The model under review builds one solid part; all positions refer to its coordinate system, in mm. A direction names the side the tool comes from. Give positions to 0.01 mm unless a question says otherwise; leave off trailing zeros. Write each loop counter-clockwise with the first axis right and the second up, starting at its lowest first coordinate (ties: lowest second). Pieces come first, ordered by that corner, then holes. Notation, with made-up numbers: (-12, -4.5) - (11, -4.5) arc R28 cw to (11, 17.5) - close; hole circle Ø4 at (-16, 89). An arc over 180 degrees is marked (long way). Write item = value, one per line.
```python
from build123d import *

# Parameters (mm, degrees)
ESQUISSE4_R             = 1.6
ENL_V_MAT_EXTRU_1_DEPTH = 10
ESQUISSE6_W             = 2.893423418
ESQUISSE6_H             = 5.635783234
ENL_V_MAT_EXTRU_3_DEPTH = 5.5


with BuildPart() as part:
    # Esquisse2 → Révolution1 (revolve)
    with BuildSketch(Plane.XY, mode=Mode.PRIVATE) as r_volution1_sk:
        Polygon((-100.191044353, 30), (-104.196152423, 30), (-104.691044353, 33.218828512), (-104.691044353, 102), (-103.641044353, 102), (-103.641044353, 119.622500925), (-101.691044353, 123), (-100.191044353, 123), align=None)
    revolve(r_volution1_sk.sketch.rotate(Axis((-100.191044353, 30, 0), (0, 1, 0)), 270), axis=Axis((-100.191044353, 30, 0), (0, 1, 0)))

    # Esquisse4 → Enlèv. mat.-Extru.1 (cut)
    with BuildSketch(Plane.XZ.offset(-30)):
        with Locations(Location((-100.191044353, 0, 0), (0, 0, 270))):
            Circle(ESQUISSE4_R)
    extrude(amount=-ENL_V_MAT_EXTRU_1_DEPTH, mode=Mode.SUBTRACT)

    # Esquisse6 → Enlèv. mat.-Extru.3 (cut, symmetric)
    with BuildSketch(Plane.XY):
        with Locations((-103.637756062, 109.817891617)):
            Rectangle(ESQUISSE6_W, ESQUISSE6_H)
        with Locations((-96.744332644, 109.817891617)):
            Rectangle(ESQUISSE6_W, ESQUISSE6_H)
    extrude(amount=ENL_V_MAT_EXTRU_3_DEPTH, both=True, mode=Mode.SUBTRACT)


solid = part.part
```
1. Draft analysis for pull direction X (two halves, no side actions). For faces 1 (the cylindrical face through (-101.61, 34.93, -0.74)), 2 (the flat face through (-102.191, 110, 0)), 3 (the flat face through (-98.191, 110, 0)), state which applies: +X half, -X half, draft (parallel to the pull), parting line (faces both ways), or undercut.
Findings below:
face_1 = undercut
face_2 = -X half
face_3 = +X half
2. Take a section at B-B on y = 68. Give the boundary of the cut face in (x, z), and give its area (3 significant figures).
Findings below:
outline = circle Ø9 at (-100.19, 0)
area = 63.6 mm²
3. Take a section at A-A on z = 0. Give the boundary of the cut face in (x, y), and give its area (3 significant figures).
Findings below:
outline = (-104.69, 33.22) - (-104.2, 30) - (-101.79, 30) - (-101.79, 40) - (-98.59, 40) - (-98.59, 30) - (-96.19, 30) - (-95.69, 33.22) - (-95.69, 102) - (-96.74, 102) - (-96.74, 107) - (-98.19, 107) - (-98.19, 112.64) - (-96.74, 112.64) - (-96.74, 119.62) - (-98.69, 123) - (-101.69, 123) - (-103.64, 119.62) - (-103.64, 112.64) - (-102.19, 112.64) - (-102.19, 107) - (-103.64, 107) - (-103.64, 102) - (-104.69, 102) - close
area = 736 mm²
4. Machinability: for faces 4 (the flat face through (-98, 107, 0)), 5 (the flat face through (-103, 112.636, 0)), 6 (the flat face through (-98, 102, -3)), which of the approach directions +Z, -Z, +X, -X, +Y, -Y give a long, thin tool a straight path to every point of the face, cutting with its end or side? Answer none if there is none.
Findings below:
face_4 = +Z, -Z, +X
face_5 = +Z, -Z, -X
face_6 = +Y
5. For line 1 (X direction, y = 36.75, z = 0); line 2 (Y direction, x = -103, z = -0.5); line 3 (Z direction, x = -100.25, y = 116), list the stretches that pass through material, from the lowest coordinate up. Write a range as from..to.
Findings below:
line_1 = -104.69..-101.79, -98.59..-95.69
line_2 = 30..107, 112.64..120.66
line_3 = -3.45..3.45
6. Insertion check: P1, Ø1.6, axis at x = -103, z = 0, coming from the +Y side; P2, Ø2, axis at x = -101.5, y = 104, coming from the -Z side; P3, Ø1, axis at x = -99.5, z = 0.5, coming from the -Y side. Each pin has a flat end and moves straight along its axis. Give the tip position at first contact, or say it passes through.
Findings below:
P1 = 122.12
P2 = -3.44
P3 = 40
